The model under review builds one solid part; all positions refer to its coordinate system, in mm. A direction names the side the tool comes from. Coordinates: 2 decimals unless noted, no trailing zeros. Loops run counter-clockwise (first coordinate to the right, second up) from the corner with the lowest first, then second, coordinate; pieces in that order, holes last. Notation, with made-up numbers: M -24,27 L 31,27 A21 ccw 31,32 Z; hole C 27.25,59.25 d3. An arc over 180 degrees is marked long. Use CSV: the item, a comma, the result in double quotes. Start each with the question number.
1. Draft analysis for pull direction Z (two halves, no side actions). For faces 1 (the cylindrical face through (-2.647, -15.653, 38.984)), 2 (the cylindrical face through (-14.71, -16.1, -16.21)), 3 (the flat face through (-43, -12.689, 53)), 4 (the flat face through (-10, -16, 54.563)), state which applies: +Z half, -Z half, draft (parallel to the pull), parting line (faces both ways), or undercut.
2. Add section B-B, the plane y = -5.5. State how many separate pieces and enclosed holes the cut face has, then the cut area to 3 significant figures.
3. Add section D-D, the plane z = -14.5. Write out the cut boundary in (x, y), then the cut area to 3 significant figures.
4. Tool access review of faces 5 (the flat face through (-13, -17.851, 53)), 6 (the flat face through (-47.472, -16, 14)): name each direction out of +Z, -Z, +X, -X, +Y, -Y from which nothing blocks a thin tool from reaching the whole face with its end or side.
5. For L1, parallel to Z at x = -7, y = -3.5; L2, parallel to Z at x = -10, y = -22; L3, parallel to X at y = -30, z = 15.5, list the stretches that pass through material, from the lowest coordinate up.
6. Add section A-A, the plane z = 17.5. Write out the cut boundary in (x, y), then the cut area to 3 significant figures.
7. Clearance check with a flat-ended pin moving along its axis: P1, Ø11, axis at x = -9.37, z = -12.11, coming from the +Y side. State where the tip first meets the part, or that it passes through.
from build123d import *

# Parameters (mm, degrees)
F0_W      = 76.2
F0_H      = 76.1999971091
F1_DEPTH  = 31.75
F2_R      = 6.731
F3_DEPTH  = 50.8
F5_R      = 6.731
F6_DEPTH  = 31.75
F7_DEPTH  = 31.751
F8_R      = 6.731
F9_DEPTH  = 31.751
F10_R     = 6.731
F11_DEPTH = 31.751
F12_R     = 6.731
F13_DEPTH = 31.751
F14_R     = 6.731
F15_DEPTH = 31.751
F16_R     = 6.731
F17_DEPTH = 31.751
F18_R     = 6.731
F19_DEPTH = 31.751
F20_W     = 76.2
F20_H     = 31.75
F20_W_2   = 1.036552576
F20_H_2   = 8.9190371367
F21_DEPTH = 3.175


with BuildPart() as f1:
    # F0 (on Front) → F1 (new body)
    with BuildSketch(Plane.XZ):
        with Locations((-9.3718003482, 13.2883749902)):
            Rectangle(F0_W, F0_H)
    extrude(amount=F1_DEPTH)

    # F2 (on face) → F3 (cut)
    with BuildSketch(Plane.XZ.offset(31.75)):
        with Locations((-9.3718003482, 13.2883735448)):
            Circle(F2_R)
    extrude(amount=-F3_DEPTH, mode=Mode.SUBTRACT)

    # F5 (on face) → F6 (cut)
    with BuildSketch(Plane.XZ.offset(31.75)):
        with Locations((16.0281996518, 38.6883735448)):
            Circle(F5_R)
    extrude(amount=-F6_DEPTH, mode=Mode.SUBTRACT)

    # F5 (on face) → F7 (cut, through all)
    with BuildSketch(Plane.XZ.offset(31.75)):
        with Locations((16.0281996518, 13.2883735448)):
            Circle(F5_R)
    extrude(amount=-F7_DEPTH, mode=Mode.SUBTRACT)

    # F8 (on face) → F9 (cut, through all)
    with BuildSketch(Plane(origin=(0, 0, 0), x_dir=(-1, 0, 0), z_dir=(0, 1, 0))):
        with Locations((9.3718003482, 38.6883735448)):
            Circle(F8_R)
    extrude(amount=-F9_DEPTH, mode=Mode.SUBTRACT)

    # F10 (on face) → F11 (cut, through all)
    with BuildSketch(Plane.XZ.offset(31.75)):
        with Locations((-34.7718003482, 38.6883735448)):
            Circle(F10_R)
    extrude(amount=-F11_DEPTH, mode=Mode.SUBTRACT)

    # F12 (on face) → F13 (cut, through all)
    with BuildSketch(Plane.XZ.offset(31.75)):
        with Locations((-34.7718003482, 13.2883735448)):
            Circle(F12_R)
    extrude(amount=-F13_DEPTH, mode=Mode.SUBTRACT)

    # F14 (on face) → F15 (cut, through all)
    with BuildSketch(Plane.XZ.offset(31.75)):
        with Locations((-34.7718003482, -12.1116235643)):
            Circle(F14_R)
    extrude(amount=-F15_DEPTH, mode=Mode.SUBTRACT)

    # F16 (on face) → F17 (cut, through all)
    with BuildSketch(Plane.XZ.offset(31.75)):
        with Locations((-9.3718003482, -12.1116235643)):
            Circle(F16_R)
    extrude(amount=-F17_DEPTH, mode=Mode.SUBTRACT)

    # F18 (on face) → F19 (cut, through all)
    with BuildSketch(Plane.XZ.offset(31.75)):
        with Locations((16.0281996518, -12.1116235643)):
            Circle(F18_R)
    extrude(amount=-F19_DEPTH, mode=Mode.SUBTRACT)

    # F20 (on face) → F21 (join)
    with BuildSketch(Plane.XY.offset(51.3883735448)):
        with Locations((-9.3718003482, -15.875)):
            Rectangle(F20_W, F20_H)
        Polygon((-40.9612769216, -12.6892459309), (-40.9612769216, -20.686903), (-41.9978294976, -20.686903), (-41.9978294976, -12.6892459309), (-44.822484069, -12.6892459309), (-44.822484069, -11.7678658633), (-38.1366223502, -11.7678658633), (-38.1366223502, -12.6892459309), align=None, mode=Mode.SUBTRACT)
        with Locations((-36.2753174892, -16.2273844317)):
            Rectangle(F20_W_2, F20_H_2, mode=Mode.SUBTRACT)
        with BuildLine():
            add(Edge.make_bspline(
                [(-27.46657267, -13.0425717618), (-28.4797003289, -12.5682171932), (-29.4928279879, -12.5682171932)],
                knots=[0, 0, 0, 1, 1, 1], degree=2))
            add(Edge.make_bspline(
                [(-29.4928279879, -12.5682171932), (-30.9627415279, -12.5682171932), (-31.8138468445, -13.5471835149)],
                knots=[0, 0, 0, 1, 1, 1], degree=2))
            add(Edge.make_bspline(
                [(-31.8138468445, -13.5471835149), (-32.6649521611, -14.5261498367), (-32.6649521611, -16.2283604699)],
                knots=[0, 0, 0, 1, 1, 1], degree=2))
            add(Edge.make_bspline(
                [(-32.6649521611, -16.2283604699), (-32.6649521611, -17.977420937), (-31.8441040289, -18.9329623418)],
                knots=[0, 0, 0, 1, 1, 1], degree=2))
            add(Edge.make_bspline(
                [(-31.8441040289, -18.9329623418), (-31.0232558967, -19.8885037466), (-29.5045404464, -19.8885037466)],
                knots=[0, 0, 0, 1, 1, 1], degree=2))
            add(Edge.make_bspline(
                [(-29.5045404464, -19.8885037466), (-28.5714479204, -19.8885037466), (-27.3748250785, -19.5527466033)],
                knots=[0, 0, 0, 1, 1, 1], degree=2))
            Line((-27.3748250785, -19.5527466033), (-27.3748250785, -20.4604621359))
            add(Edge.make_bspline(
                [(-27.3748250785, -20.4604621359), (-28.3020613753, -20.8098838141), (-29.662658636, -20.8098838141)],
                knots=[0, 0, 0, 1, 1, 1], degree=2))
            add(Edge.make_bspline(
                [(-29.662658636, -20.8098838141), (-31.6323037379, -20.8098838141), (-32.7030176512, -19.6132609722)],
                knots=[0, 0, 0, 1, 1, 1], degree=2))
            add(Edge.make_bspline(
                [(-32.7030176512, -19.6132609722), (-33.7737315644, -18.4166381302), (-33.7737315644, -16.214695935)],
                knots=[0, 0, 0, 1, 1, 1], degree=2))
            add(Edge.make_bspline(
                [(-33.7737315644, -16.214695935), (-33.7737315644, -14.8365299865), (-33.258383391, -13.7999774106)],
                knots=[0, 0, 0, 1, 1, 1], degree=2))
            add(Edge.make_bspline(
                [(-33.258383391, -13.7999774106), (-32.7430352176, -12.7634248346), (-31.7699251252, -12.2022028655)],
                knots=[0, 0, 0, 1, 1, 1], degree=2))
            add(Edge.make_bspline(
                [(-31.7699251252, -12.2022028655), (-30.7968150327, -11.6409808964), (-29.479163453, -11.6409808964)],
                knots=[0, 0, 0, 1, 1, 1], degree=2))
            add(Edge.make_bspline(
                [(-29.479163453, -11.6409808964), (-28.0775725876, -11.6409808964), (-27.0273554768, -12.1524249169)],
                knots=[0, 0, 0, 1, 1, 1], degree=2))
            Line((-27.0273554768, -12.1524249169), (-27.46657267, -13.0425717618))
        make_face(mode=Mode.SUBTRACT)
        Polygon((-19.4376823782, -12.6892459309), (-19.4376823782, -20.686903), (-20.4742349542, -20.686903), (-20.4742349542, -12.6892459309), (-23.2988895256, -12.6892459309), (-23.2988895256, -11.7678658633), (-16.6130278068, -11.7678658633), (-16.6130278068, -12.6892459309), align=None, mode=Mode.SUBTRACT)
        Polygon((-8.5899937443, -20.686903), (-9.6636357721, -20.686903), (-10.7743672518, -17.8505359701), (-14.3486191663, -17.8505359701), (-15.4456861111, -20.686903), (-16.4959032219, -20.686903), (-12.9704532178, -11.7307764115), (-12.0978750606, -11.7307764115), align=None, mode=Mode.SUBTRACT)
        with BuildLine():
            add(Edge.make_bspline(
                [(-1.5195729719, -13.0425717618), (-2.5327006309, -12.5682171932), (-3.5458282899, -12.5682171932)],
                knots=[0, 0, 0, 1, 1, 1], degree=2))
            add(Edge.make_bspline(
                [(-3.5458282899, -12.5682171932), (-5.0157418298, -12.5682171932), (-5.8668471464, -13.5471835149)],
                knots=[0, 0, 0, 1, 1, 1], degree=2))
            add(Edge.make_bspline(
                [(-5.8668471464, -13.5471835149), (-6.717952463, -14.5261498367), (-6.717952463, -16.2283604699)],
                knots=[0, 0, 0, 1, 1, 1], degree=2))
            add(Edge.make_bspline(
                [(-6.717952463, -16.2283604699), (-6.717952463, -17.977420937), (-5.8971043308, -18.9329623418)],
                knots=[0, 0, 0, 1, 1, 1], degree=2))
            add(Edge.make_bspline(
                [(-5.8971043308, -18.9329623418), (-5.0762561986, -19.8885037466), (-3.5575407483, -19.8885037466)],
                knots=[0, 0, 0, 1, 1, 1], degree=2))
            add(Edge.make_bspline(
                [(-3.5575407483, -19.8885037466), (-2.6244482223, -19.8885037466), (-1.4278253804, -19.5527466033)],
                knots=[0, 0, 0, 1, 1, 1], degree=2))
            Line((-1.4278253804, -19.5527466033), (-1.4278253804, -20.4604621359))
            add(Edge.make_bspline(
                [(-1.4278253804, -20.4604621359), (-2.3550616772, -20.8098838141), (-3.7156589379, -20.8098838141)],
                knots=[0, 0, 0, 1, 1, 1], degree=2))
            add(Edge.make_bspline(
                [(-3.7156589379, -20.8098838141), (-5.6853040399, -20.8098838141), (-6.7560179531, -19.6132609722)],
                knots=[0, 0, 0, 1, 1, 1], degree=2))
            add(Edge.make_bspline(
                [(-6.7560179531, -19.6132609722), (-7.8267318663, -18.4166381302), (-7.8267318663, -16.214695935)],
                knots=[0, 0, 0, 1, 1, 1], degree=2))
            add(Edge.make_bspline(
                [(-7.8267318663, -16.214695935), (-7.8267318663, -14.8365299865), (-7.3113836929, -13.7999774106)],
                knots=[0, 0, 0, 1, 1, 1], degree=2))
            add(Edge.make_bspline(
                [(-7.3113836929, -13.7999774106), (-6.7960355196, -12.7634248346), (-5.8229254271, -12.2022028655)],
                knots=[0, 0, 0, 1, 1, 1], degree=2))
            add(Edge.make_bspline(
                [(-5.8229254271, -12.2022028655), (-4.8498153346, -11.6409808964), (-3.532163755, -11.6409808964)],
                knots=[0, 0, 0, 1, 1, 1], degree=2))
            add(Edge.make_bspline(
                [(-3.532163755, -11.6409808964), (-2.1305728895, -11.6409808964), (-1.0803557787, -12.1524249169)],
                knots=[0, 0, 0, 1, 1, 1], degree=2))
            Line((-1.0803557787, -12.1524249169), (-1.5195729719, -13.0425717618))
        make_face(mode=Mode.SUBTRACT)
        Polygon((6.5093173199, -12.6892459309), (6.5093173199, -20.686903), (5.4727647439, -20.686903), (5.4727647439, -12.6892459309), (2.6481101725, -12.6892459309), (2.6481101725, -11.7678658633), (9.3339718913, -11.7678658633), (9.3339718913, -12.6892459309), align=None, mode=Mode.SUBTRACT)
        with BuildLine():
            add(Edge.make_bspline(
                [(17.3394372661, -12.8473641204), (18.4189355232, -14.0674118793), (18.4189355232, -16.214695935)],
                knots=[0, 0, 0, 1, 1, 1], degree=2))
            add(Edge.make_bspline(
                [(18.4189355232, -16.214695935), (18.4189355232, -18.3561237614), (17.3355331133, -19.5830037877)],
                knots=[0, 0, 0, 1, 1, 1], degree=2))
            add(Edge.make_bspline(
                [(17.3355331133, -19.5830037877), (16.2521307034, -20.8098838141), (14.3254312825, -20.8098838141)],
                knots=[0, 0, 0, 1, 1, 1], degree=2))
            add(Edge.make_bspline(
                [(14.3254312825, -20.8098838141), (12.3557861805, -20.8098838141), (11.2850722673, -19.6044766283)],
                knots=[0, 0, 0, 1, 1, 1], degree=2))
            add(Edge.make_bspline(
                [(11.2850722673, -19.6044766283), (10.2143583541, -18.3990694425), (10.2143583541, -16.2029834765)],
                knots=[0, 0, 0, 1, 1, 1], degree=2))
            add(Edge.make_bspline(
                [(10.2143583541, -16.2029834765), (10.2143583541, -14.0244661982), (11.2880003819, -12.8258912799)],
                knots=[0, 0, 0, 1, 1, 1], degree=2))
            add(Edge.make_bspline(
                [(11.2880003819, -12.8258912799), (12.3616424098, -11.6273163615), (14.337143741, -11.6273163615)],
                knots=[0, 0, 0, 1, 1, 1], degree=2))
            add(Edge.make_bspline(
                [(14.337143741, -11.6273163615), (16.259939009, -11.6273163615), (17.3394372661, -12.8473641204)],
                knots=[0, 0, 0, 1, 1, 1], degree=2))
        make_face(mode=Mode.SUBTRACT)
        Polygon((25.3780879399, -19.7596667032), (25.3780879399, -20.686903), (20.4061493129, -20.686903), (20.4061493129, -11.7678658633), (25.3780879399, -11.7678658633), (25.3780879399, -12.6892459309), (21.4427018888, -12.6892459309), (21.4427018888, -15.5627024126), (25.1399346174, -15.5627024126), (25.1399346174, -16.4782262509), (21.4427018888, -16.4782262509), (21.4427018888, -19.7596667032), align=None, mode=Mode.SUBTRACT)
    extrude(amount=F21_DEPTH)


solid = f1.part
Computed:
1,face 1,"undercut"
1,face 2,"undercut"
1,face 3,"draft"
1,face 4,"+Z half"
2,separate pieces,"1"
2,enclosed holes,"9"
2,area,"4,770 mm^2"
3,outline,"M -47.47,-31.75 L -41.06,-31.75 L -41.06,0 L -47.47,0 Z; M -28.48,-31.75 L -15.66,-31.75 L -15.66,0 L -28.48,0 Z; M -3.08,-31.75 L 9.74,-31.75 L 9.74,0 L -3.08,0 Z; M 22.32,-31.75 L 28.73,-31.75 L 28.73,0 L 22.32,0 Z"
3,area,"1,220 mm^2"
4,face 5,"+Z"
4,face 6,"+Z, -Z, -X, +Y, -Y"
5,L1,"z = -24.81 to -18.41, -5.81 to 6.99, 19.59 to 32.39, 44.99 to 54.56"
5,L2,"z = -24.81 to -18.81, -5.41 to 6.59, 19.99 to 31.99, 45.39 to 54.56"
5,L3,"x = -47.47 to -41.13, -28.41 to -15.73, -3.01 to 9.67, 22.39 to 28.73"
6,outline,"M -47.47,-31.75 L -40.02,-31.75 L -40.02,0 L -47.47,0 Z; M -29.52,-31.75 L -14.62,-31.75 L -14.62,0 L -29.52,0 Z; M -4.12,-31.75 L 10.78,-31.75 L 10.78,0 L -4.12,0 Z; M 21.28,-31.75 L 28.73,-31.75 L 28.73,0 L 21.28,0 Z"
6,area,"1,420 mm^2"
7,P1,"passes through"
